Solid Edge part; units mm, degrees
sketch "Sketch1" plane through (0, 0, 0) normal (0, -1, 0) x (1, 0, 0)
  line L0 (52, 38.5) -> (52, -11.5)
  line L1 (52, 38.5) -> (-4.6369, 29.6395)
  arc A0 (52, -11.5) -> (17.1896, -24.587) centre (60.1635, -86.0544) ccw
  arc A1 (17.1896, -24.587) -> (-4.6369, 29.6395) centre (0, 0) cw
  dimension "D1" = 52
extrude "Protrusion1" add sketch "Sketch1" against normal blind 15
sketch "Sketch2" plane through (11, 0, 4.25) normal (0, -1, 0) x (0.9879828, 0, 0.1545642)
  circle A0 centre (-11.5247, -2.4987) radius 20
extrude "VaciadoExtruido_1" cut sketch "Sketch2" against normal blind 3
sketch "Sketch3" plane through (0, 3, 0) normal (0, -1, 0) x (1, 0, 0)
  line L0 (6, -6) -> (-6, -6)
  line L1 (-6, -6) -> (-6, 6)
  line L2 (-6, 6) -> (6, 6)
  line L3 (6, 6) -> (6, -6)
  dimension "D1" = 6
  dimension "D2" = 6
extrude "VaciadoExtruido_2" cut sketch "Sketch3" against normal blind 9
sketch "Sketch4" plane through (0, 12, 0) normal (0, -1, 0) x (1, 0, 0)
  circle A0 centre (0, 0) radius 3.2
extrude "Cutout1" cut sketch "Sketch4" against normal through all
hole "Agujero_1" at (-13, 15, 0) direction (0, -1, 0) diameter 4.5 end up to next counterbore diameter 8 counterbore depth 7
pattern_circular "Pattern1" count 6 over 360 about axis through (0, 15, 0) along (0, 1, 0) of "Agujero_1"
hole "Agujero_7" at (52, 7.5, 28.5) direction (-1, 0, 0) diameter 4.917 depth 12 tip angle 118 thread major 6 thread length 10
hole "Hole6" at (52, 7.5, 13.5) direction (-1, 0, 0) diameter 4.917 depth 12 tip angle 118 thread major 6 thread length 10
hole "Hole7" at (52, 7.5, -1.5) direction (-1, 0, 0) diameter 4.917 depth 12 tip angle 118 thread major 6 thread length 10
properties part number "1976-1400-001" material "Aluminio, 7075-T6"
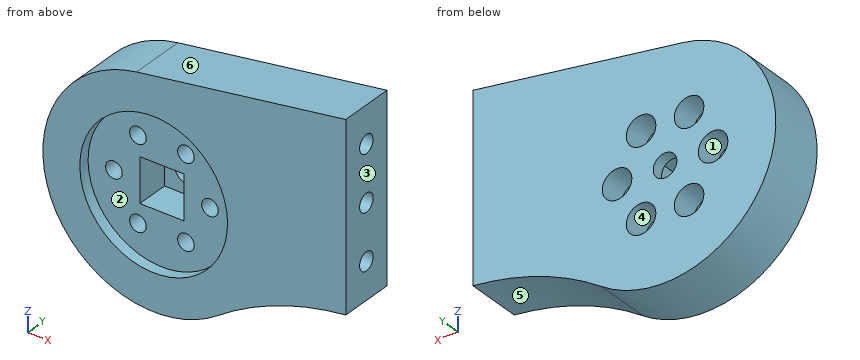
Part model, mm, in its own coordinate system. Face numbers are marked on the shaded views. A direction names the side the tool comes from. Coordinates: 2 decimals unless noted, no trailing zeros. Write each loop counter-clockwise with the first axis right and the second up, starting at its lowest first coordinate (ties: lowest second). Pieces come first, ordered by that corner, then holes.
Item 1: Probe line 1 (Y direction, x = 47.25, z = 28.5); line 2 (Z direction, x = 46, y = 6.25); line 3 (Z direction, x = 48.5, y = 7.5). List the from-to ranges inside material, lowest first.
Item 2: Mould opens along X. For the marked faces 4, 5 and 6 say: released by +X, released by -X, zero draft, split by the parting line, or undercut.
Item 3: Pin check, flat tips, straight feed: pin 1 (2 mm diameter, centred on x = -20.5, y = 13, fed in from -Z); pin 2 (2 mm diameter, centred on x = 0, z = 21.5, fed in from -Y); pin 3 (7 mm diameter, centred on x = -13, z = 0, fed in from -Y); pin 4 (2.5 mm diameter, centred on x = 6.5, z = -11.26, fed in from -Y). Stop position of each tip, or through.
Item 4: Slice it at C-C (x = 13). Write the cut outline in (y, z), and give its area (3 significant figures).
Item 5: Which spindle directions (+Z, -Z, +X, -X, +Y, -Y) get a long thin tool onto all of the face, cutting with end or side? Do the marked faces 1, 2 and 3. Say none if no direction does.
Item 6: Slice it at B-B (z = 0). Count the separate pieces of the cut face and the enclosed holes in it, and give its area (3 significant figures).
Item 7: Slice it at A-A (x = 0). Write the cut outline in (y, z), and give its area (3 significant figures).
Results found:
1. line 1: y = 0 to 5.04, 9.96 to 15
1. line 2: z = -12.4 to -3.62, 0.62 to 11.38, 15.62 to 26.38, 30.62 to 37.56
1. line 3: z = -11.97 to -3.96, 0.96 to 11.04, 15.96 to 26.04, 30.96 to 37.95
2. face 4: undercut
2. face 5: released by +X
2. face 6: released by -X
3. pin 1: stops at z = -22.8
3. pin 2: stops at y = 0
3. pin 3: stops at y = 3
3. pin 4: passes through
4. outline: (0, -27.04) - (15, -27.04) - (15, -4) - (8, -4) - (8, -2.25) - (3, -2.25) - (3, -15.2) - (0, -15.2) - close; (0, 15.2) - (3, 15.2) - (3, 2.25) - (8, 2.25) - (8, 4) - (15, 4) - (15, 32.4) - (0, 32.4) - close
4. area: 722 mm2
5. face 1: +Y
5. face 2: -Y
5. face 3: +Z, -Z, +X, +Y, -Y
6. separate pieces: 4
6. enclosed holes: 0
6. area: 778 mm2
7. outline: (0, -30) - (15, -30) - (15, -3.2) - (12, -3.2) - (12, -6) - (3, -6) - (3, -20) - (0, -20) - close; (0, 20) - (3, 20) - (3, 6) - (12, 6) - (12, 3.2) - (15, 3.2) - (15, 30.36) - (0, 30.36) - close
7. area: 658 mm2
